Check sheet for the modelled part. Datum: model origin and axes. Units: mm. A direction names the side the tool comes from. Round coordinates to 2 decimals unless told otherwise and drop trailing zeros. Write each loop counter-clockwise with the first axis right and the second up, starting at its lowest first coordinate (ties: lowest second). Pieces come first, ordered by that corner, then holes. Notation, with made-up numbers: (27, 55) -> (63, 55) arc R21 cw to (63, 84) -> close; hole circle Ø2 at (51, 34). An arc over 180 degrees is marked (long way). Write item = value, one per line.
from build123d import *

# Parameters (mm, degrees)
SKETCH_2_R               = 16.8
EXTRUDE_1_DEPTH          = 18
SKETCH_4_R               = 4.3
CUT_EXTRUDE_1_DEPTH      = 19
CHAMFER_1_SIZE           = 2
PATTERN_CIRCULAR_1_COUNT = 4
SKETCH_8_R               = 5.3
SKETCH_8_R_2             = 4.3
EXTRUDE_1_2_DEPTH        = 2
SKETCH_9_R               = 5.3
SKETCH_9_R_2             = 4.8
CUT_EXTRUDE_1_2_DEPTH    = 0.5
SKETCH_10_R              = 16.8
SKETCH_10_R_2            = 15.8
CUT_EXTRUDE_2_DEPTH      = 1
PATTERN_CIRCULAR_2_COUNT = 4


with BuildPart() as part:
    # Sketch 2 → Extrude 1 (new body)
    with BuildSketch(Plane(origin=(0, 0, 0), x_dir=(1, 0, 0), z_dir=(0, 1, 0))):
        Circle(SKETCH_2_R)
    extrude(amount=EXTRUDE_1_DEPTH)

    # Sketch 4 → Cut-Extrude 1 (cut, through all)
    with BuildSketch(Plane(origin=(0, 18, 0), x_dir=(1, 0, 0), z_dir=(0, 1, 0))):
        Circle(SKETCH_4_R)
    extrude(amount=-CUT_EXTRUDE_1_DEPTH, mode=Mode.SUBTRACT)

    # Chamfer 1
    chamfer_1_edges = [part.edges().sort_by_distance(p)[0] for p in [
        (-16.8, 18, 0),
    ]]
    chamfer(chamfer_1_edges, length=CHAMFER_1_SIZE)

    # Sketch 7 → Hole Wizard M2.5 _1 (revolve, cut)
    with BuildSketch(Plane(origin=(0, 18, -8), x_dir=(0, 0, 1), z_dir=(1, 0, 0))):
        Polygon((0, 0), (0, 4.615882135), (1.025, 4), (1.025, 0), align=None)
    hole_wizard_m2_5_1 = revolve(axis=Axis((0, 24.35, -8), (0, -1, 0)), mode=Mode.SUBTRACT)

    # Pattern Circular 1: Hole Wizard M2.5 _1 ×4 about axis
    pattern_circular_1_axis = Axis((0, 0, 0), (0, 1, 0))
    for i in range(1, PATTERN_CIRCULAR_1_COUNT):
        add(hole_wizard_m2_5_1.rotate(pattern_circular_1_axis, i * 360 / PATTERN_CIRCULAR_1_COUNT), mode=Mode.SUBTRACT)

    # Sketch 8 → Extrude 1 2 (add)
    with BuildSketch(Plane.XZ):
        Circle(SKETCH_8_R)
        Circle(SKETCH_8_R_2, mode=Mode.SUBTRACT)
    extrude(amount=EXTRUDE_1_2_DEPTH)

    # Sketch 9 → Cut-Extrude 1 2 (cut)
    with BuildSketch(Plane.XZ.offset(2)):
        Circle(SKETCH_9_R)
        Circle(SKETCH_9_R_2, mode=Mode.SUBTRACT)
    extrude(amount=-CUT_EXTRUDE_1_2_DEPTH, mode=Mode.SUBTRACT)

    # Sketch 10 → Cut-Extrude 2 (cut)
    with BuildSketch(Plane.XZ):
        Circle(SKETCH_10_R)
        Circle(SKETCH_10_R_2, mode=Mode.SUBTRACT)
    extrude(amount=-CUT_EXTRUDE_2_DEPTH, mode=Mode.SUBTRACT)

    # Sketch 12 → Hole Wizard M2.5 _2 (revolve, cut)
    with BuildSketch(Plane(origin=(11, 0, 0), x_dir=(0, 0, -1), z_dir=(1, 0, 0))):
        Polygon((0, 0), (0, 4.615882135), (1.025, 4), (1.025, 0), align=None)
    hole_wizard_m2_5_2 = revolve(axis=Axis((11, -6.35, 0), (0, 1, 0)), mode=Mode.SUBTRACT)

    # Pattern Circular 2: Hole Wizard M2.5 _2 ×4 about axis
    pattern_circular_2_axis = Axis((0, 0, 0), (0, 1, 0))
    for i in range(1, PATTERN_CIRCULAR_2_COUNT):
        add(hole_wizard_m2_5_2.rotate(pattern_circular_2_axis, i * 360 / PATTERN_CIRCULAR_2_COUNT), mode=Mode.SUBTRACT)


solid = part.part
(1) Release check for a two-part mould opening along Z. For faces 4 (the flat face through (7, 0, 0)), 5 (the conical face through (-10.85, 4.509, 0.096)), 6 (the cylindrical face through (16.024, 8.395, -5.046)) record: pulls with the +Z half, pulls with the -Z half, needs draft (parallel to the pull), parting line crosses it, or undercut.
Worked answers:
face_4 = needs draft
face_5 = undercut
face_6 = parting line crosses it
(2) Go/stop test with flat-tipped pins: P1, Ø5, axis at y = 13.5, z = 9.5, coming from the -X side; P2, Ø10, axis at x = -5.5, y = 3, coming from the -Z side; P3, Ø1.5, axis at y = 15, z = -7, coming from the +X side. Record where each tip stops, or that it passes through.
Worked answers:
P1 = -15.27
P2 = -16.79
P3 = 15.59
(3) Sectioned sample at A-A on y = 11.5. Enter the section's corners in (x, z).
Worked answers:
outline = circle Ø33.6 at (0, 0); hole circle Ø8.6 at (0, 0)
(4) Access from +Z, -Z, +X, -X, +Y, -Y to the whole of each face (thin tool, end or side, straight path). Record for faces 1 (the flat face through (-4, -2, 2)), 2 (the cylindrical face through (-9.024, 16.028, 0.045)), 3 (the cylindrical face through (10.31, 1.97, 0.76)).
Worked answers:
face_1 = +Z, -Z, +X, -X, -Y
face_2 = +Y
face_3 = -Y
(5) Material ranges on L1, parallel to X at y = 2.35, z = 0 (3 decimals); L2, parallel to X at y = 9.5, z = 0, recorded low to high. Write a range as [from, to].
Worked answers:
L1 = [-16.8, -12.025], [-9.975, -4.3], [4.3, 9.975], [12.025, 16.8]
L2 = [-16.8, -4.3], [4.3, 16.8]
